Could you check a few things on this model? Use its own coordinates, in mm. A direction names the side the tool comes from. Give positions to 0.01 mm unless a question says otherwise; leave off trailing zeros. Order: outer loops, then holes, each group sorted by start corner. A loop starts at its lowest first (then second) coordinate and runs counter-clockwise, first axis right, second up.
(1) Will these pins go through, and if not, where does the flat tip stop? pin 1 (1 mm diameter, centred on y = 5, z = -68, fed in from -X); pin 2 (4.5 mm diameter, centred on x = -6, z = -4.5, fed in from +Y); pin 3 (2.5 mm diameter, centred on x = -13, z = -108.5, fed in from -Y).
(2) If I drill on probe 1 along Z at (x, y) = (-6, 0.7); probe 2 along Z at (x, y) = (-13, 1); probe 3 along X at (y, z) = (0.85, -108.5), over which ranges is the centre line in solid material (lowest first)?
(3) Imagine slicing it at B-B, the plane z = -115.5. Write out the boundary of the cut face in (x, y), then the cut area to 4 significant figures.
(4) Imagine slicing it at D-D, the plane y = 6. Write out the boundary of the cut face in (x, z).
(5) Imagine slicing it at A-A, the plane x = -6. Write out the boundary of the cut face in (y, z), then the cut area to 3 significant figures.
(6) If we mould it in two halves opening along Z, with no side actions, what happens to faces 3 (the flat face through (-10, 0, -59)), 4 (the flat face through (-7, 1, 0)), 5 (the cylindrical face through (-13.26, 0.76, -13.483)), 6 (the flat face through (-7, 1, -120))? For each: released by +Z, released by -Z, zero draft, split by the parting line, or undercut.
(7) On a 3-axis mill with a long thin cutter (end or side, diameter ignored), from which of +Z, -Z, +X, -X, +Y, -Y can I reach the whole of each face in a straight line? I mean faces 1 (the flat face through (-1.5, 6, -59)), 2 (the cylindrical face through (-13.26, 0.76, -110.483)). Say none if no direction works.
(8) Imagine slicing it at C-C, the plane z = -74. Write out the boundary of the cut face in (x, y), then the cut area to 4 significant figures.
Autodesk Inventor part; units mm, degrees
ref_plane "YZ Plane" through (0, 0, 0) normal (1, 0, 0) x (0, 1, 0)
ref_plane "XZ Plane" through (0, 0, 0) normal (0, 1, 0) x (-1, 0, 0)
ref_plane "XY Plane" through (0, 0, 0) normal (0, 0, 1) x (1, 0, 0)
sketch "Sketch1" plane through (0, 0, 0) normal (0, 1, 0) x (-1, 0, 0)
  line L0 (0, 0) -> (20, 0)
  line L1 (20, 0) -> (20, -120)
  line L2 (20, -120) -> (0, -120)
  line L3 (0, -120) -> (0, 0)
  dimension "d0" = 20
  dimension "d1" = 120
extrude "Extrusion1" add sketch "Sketch1" along normal blind 1.5
sketch "Sketch2" plane through (0, 0, 0) normal (0, -1, 0) x (1, 0, 0)
  line L0 (0, 0) -> (-1.5, 0)
  line L1 (-1.5, 0) -> (-1.5, -120)
  line L2 (-1.5, -120) -> (0, -120)
  line L3 (0, -120) -> (0, 0)
  dimension "d4" = 1.5
  dimension "d5" = 120
extrude "Extrusion2" add sketch "Sketch2" against normal blind 10
sketch "Sketch3" plane through (0, 1.5, 0) normal (0, 1, 0) x (1, 0, 0)
  line L0 (-20, 120) -> (-20, 0)
  line L1 (-20, 120) -> (-1.5, 120)
  line L2 (-1.5, 120) -> (-1.5, 101.5)
  line L3 (-1.5, 101.5) -> (-20, 101.5)
  line L4 (-20, 101.5) -> (-20, 120)
  line L5 (-20, 0) -> (-1.5, 0)
  line L6 (-1.5, 0) -> (-1.5, 18.5)
  line L7 (-1.5, 18.5) -> (-20, 18.5)
  line L8 (-20, 18.5) -> (-20, 0)
  line L9 (-20, 101.5) -> (-13, 101.5)
  line L10 (-13, 101.5) -> (-13, 108.5)
  line L11 (-13, 108.5) -> (-20, 108.5)
  line L12 (-20, 108.5) -> (-20, 101.5)
  line L13 (-20, 101.5) -> (-6, 101.5)
  line L14 (-6, 101.5) -> (-6, 115.5)
  line L15 (-6, 115.5) -> (-20, 115.5)
  line L16 (-20, 115.5) -> (-20, 101.5)
  circle A0 centre (-6, 115.5) radius 2
  circle A1 centre (-13, 108.5) radius 2
  line L17 (-20, 18.5) -> (-13, 18.5)
  line L18 (-13, 18.5) -> (-13, 11.5)
  line L19 (-13, 11.5) -> (-20, 11.5)
  line L20 (-20, 11.5) -> (-20, 18.5)
  line L21 (-20, 18.5) -> (-6, 18.5)
  line L22 (-6, 18.5) -> (-6, 4.5)
  line L23 (-6, 4.5) -> (-20, 4.5)
  line L24 (-20, 4.5) -> (-20, 18.5)
  circle A2 centre (-13, 11.5) radius 2
  circle A3 centre (-6, 4.5) radius 2
  point P0 (0, 0)
  dimension "d8" = 18.5
  dimension "d9" = 18.5
  dimension "d10" = 18.5
  dimension "d11" = 18.5
  dimension "d12" = 7
  dimension "d13" = 7
  dimension "d14" = 14
  dimension "d15" = 14
  dimension "d16" = 4
  dimension "d17" = 4
  dimension "d18" = 7
  dimension "d19" = 7
  dimension "d20" = 14
  dimension "d21" = 14
  dimension "d22" = 4
  dimension "d23" = 4
extrude "Extrusion3" cut sketch "Sketch3" against normal blind 10 contours A0 L14 L15 | L15 L14 A0 | A1 L10 L11 | L11 L10 A1 | A2 L18 L19 | L19 L18 A2 | A3 L22 L23 | L23 L22 A3
properties part number "aluminium_profile_1"
Answer block:
1. pin 1: stops at x = -1.5
1. pin 2: stops at y = 1.5
1. pin 3: passes through
2. probe 1: z = -120 to -117.5, -113.5 to -6.5, -2.5 to 0
2. probe 2: z = -120 to -110.5, -106.5 to -13.5, -9.5 to 0
2. probe 3: x = -20 to -15, -11 to 0
3. outline: (-20, 0) - (-8, 0) - (-8, 1.5) - (-20, 1.5) - close; (-4, 0) - (0, 0) - (0, 10) - (-1.5, 10) - (-1.5, 1.5) - (-4, 1.5) - close
3. area: 36.75 mm2
4. outline: (-1.5, -120) - (0, -120) - (0, 0) - (-1.5, 0) - close
5. outline: (0, -120) - (1.5, -120) - (1.5, -117.5) - (0, -117.5) - close; (0, -113.5) - (1.5, -113.5) - (1.5, -6.5) - (0, -6.5) - close; (0, -2.5) - (1.5, -2.5) - (1.5, 0) - (0, 0) - close
5. area: 168 mm2
6. face 3: zero draft
6. face 4: released by +Z
6. face 5: undercut
6. face 6: released by -Z
7. face 1: +Z, -Z, -X, +Y
7. face 2: +Y, -Y
8. outline: (-20, 0) - (0, 0) - (0, 10) - (-1.5, 10) - (-1.5, 1.5) - (-20, 1.5) - close
8. area: 42.75 mm2
